Source: CAD feature listing. Evaluate the final solid. Frame: model axes, mm. Face numbers are marked on the shaded views. Round coordinates to 2 decimals unless told otherwise and drop trailing zeros. Order: outer loops, then holes, each group sorted by start corner. A loop starts at its lowest first (then second) coordinate and runs counter-clockwise, first axis right, second up. Notation, with made-up numbers: (-29.75, 83) -> (-22.75, 83) arc R38 cw to (-22.75, 122) -> close; hole circle Ø6 at (-2.5, 54.25). An arc over 180 degrees is marked (long way). Answer as CSV lines item,"result".
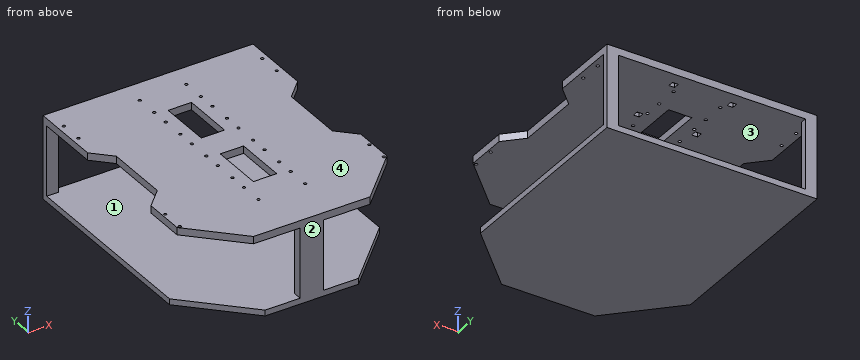
Autodesk Inventor part; units mm, degrees
ref_plane "YZ Plane" through (0, 0, 0) normal (1, 0, 0) x (0, 1, 0)
ref_plane "XZ Plane" through (0, 0, 0) normal (0, 1, 0) x (-1, 0, 0)
ref_plane "XY Plane" through (0, 0, 0) normal (0, 0, 1) x (1, 0, 0)
sketch "Boceto1" plane through (0, 0, 0) normal (0, 0, 1) x (1, 0, 0)
  line L0 (0, 0) -> (-180, 0)
  line L1 (-180, 0) -> (-180, -120)
  line L2 (-180, -120) -> (-150, -150)
  line L3 (-150, -150) -> (-150, -260)
  line L4 (-150, -260) -> (-180, -290)
  line L5 (-180, -290) -> (-180, -360)
  line L6 (-180, -360) -> (-100, -440)
  line L7 (-100, -440) -> (0, -440)
  line L8 (0, -440) -> (0, 0) construction
  line L9 (0, 0) -> (180, 0)
  line L10 (180, 0) -> (180, -120)
  line L11 (180, -120) -> (150, -150)
  line L12 (150, -150) -> (150, -260)
  line L13 (150, -260) -> (180, -290)
  line L14 (180, -290) -> (180, -360)
  line L15 (180, -360) -> (100, -440)
  line L16 (100, -440) -> (0, -440)
  dimension "d0" = 120
  dimension "d1" = 70
  dimension "d2" = 110
  dimension "d3" = 180
  dimension "d8" = 100
  dimension "d9" = 80
  dimension "d13" = 150
  dimension "d17" = 80
  dimension "d18" = 30
  dimension "d19" = 30
extrude "Extrusión1" add sketch "Boceto1" along normal mid plane 12.55
sketch "Boceto2" plane through (0, 0, 6.275) normal (0, 0, 1) x (1, 0, 0)
  line L0 (0, 0) -> (0, -440)
  line L1 (-100, -440) -> (100, -440)
  line L2 (180, 0) -> (180, -120)
  line L3 (180, -120) -> (-179.9429, -120)
  line L4 (180, -120) -> (150, -150)
  line L5 (180, -120) -> (180, -60)
  line L6 (180, -60) -> (0, -60)
  line L7 (0, -60) -> (15, -60)
  line L8 (15, -60) -> (-15, -60)
  line L9 (180, -60) -> (170, -60)
  line L10 (170, -60) -> (170, -79.5)
  line L11 (170, -79.5) -> (170, -40.5)
  circle A0 centre (170, -40.5) radius 2.5
  circle A1 centre (170, -79.5) radius 2.5
  circle A2 centre (-170, -40.5) radius 2.5
  circle A3 centre (-170, -79.5) radius 2.5
  dimension "d20" = 60
  dimension "d22" = 30
  dimension "d23" = 10
  dimension "d25" = 39
  dimension "d26" = 5
extrude "Extrusión2" cut sketch "Boceto2" against normal blind 14.75 contours A1 | A0 | A2 | A3
sketch "Boceto3" plane through (0, 0, 6.275) normal (0, 0, 1) x (1, 0, 0)
  circle A0 centre (170, -40.5) radius 2.5
  line L0 (170, -40.5) -> (170, -60)
  line L1 (170, -60) -> (0, -60)
  line L2 (0, -60) -> (0, -130)
  line L3 (0, -130) -> (40, -130)
  line L4 (40, -130) -> (-40, -130)
  line L5 (40, -130) -> (40, -110.5)
  circle A1 centre (40, -110.5) radius 2.5
  circle A2 centre (40, -149.5) radius 2.5
  circle A3 centre (-40, -110.5) radius 2.5
  circle A4 centre (-40, -149.5) radius 2.5
  line L6 (40, -130) -> (40, -200)
  line L7 (40, -200) -> (40, -165)
  line L8 (40, -165) -> (-88.7042, -165)
  circle A5 centre (40, -219.5) radius 2.5
  circle A6 centre (40, -180.5) radius 2.5
  circle A7 centre (-40, -219.5) radius 2.5
  circle A8 centre (-40, -180.5) radius 2.5
  line L9 (40, -180.5) -> (40, -200)
  line L10 (40, -200) -> (40, -270)
  line L11 (40, -270) -> (-42.5, -270)
  line L12 (40, -270) -> (40, -235)
  line L13 (40, -235) -> (-24.3521, -235)
  circle A9 centre (40, -359.5) radius 2.5
  circle A10 centre (40, -320.5) radius 2.5
  circle A11 centre (-40, -359.5) radius 2.5
  circle A12 centre (-40, -320.5) radius 2.5
  circle A13 centre (40, -250.5) radius 2.5
  circle A14 centre (40, -289.5) radius 2.5
  circle A15 centre (-40, -250.5) radius 2.5
  circle A16 centre (-40, -289.5) radius 2.5
  line L14 (40, -165) -> (40, -95)
  line L15 (40, -95) -> (-4.3592, -95)
  circle A17 centre (40, -79.5) radius 2.5
  circle A18 centre (40, -40.5) radius 2.5
  circle A19 centre (-40, -79.5) radius 2.5
  circle A20 centre (-40, -40.5) radius 2.5
  point P0 (0, 0)
  dimension "d29" = 19.5
  dimension "d30" = 70
  dimension "d31" = 40
  dimension "d32" = 80
  dimension "d33" = 19.5
  dimension "d34" = 5
  dimension "d37" = 70
  dimension "d38" = 70
  dimension "d39" = 35
  dimension "d46" = 70
extrude "Extrusión3" cut sketch "Boceto3" against normal blind 14.75 contours A13 L10 | L10 A13 | A5 L10 | L10 A5 | A6 L6 | L6 A6 | A2 L6 | L6 A2 | L14 L5 A1 | A1 L5 L14 | A3 | A4 | A7 | A8 | A9 | A10 | A11 | A12 | A14 | A15 | A16 | A17 | A18 | A19 | A20
sketch "Boceto4" plane through (0, 0, 6.275) normal (0, 0, 1) x (1, 0, 0)
  circle A0 centre (40, -320.5) radius 2.5
  line L0 (40, -320.5) -> (180, -320.5)
  line L1 (180, -360) -> (180, -290)
  line L2 (180, -320.5) -> (175, -320.5)
  line L3 (175, -320.5) -> (175, -359.5)
  circle A1 centre (175, -320.5) radius 2.5
  circle A2 centre (175, -359.5) radius 2.5
  line L4 (-100, -440) -> (100, -440)
  line L5 (0, -440) -> (0, 0)
  circle A3 centre (-175, -320.5) radius 2.5
  circle A4 centre (-175, -359.5) radius 2.5
  dimension "d40" = 5
  dimension "d41" = 39
  dimension "d42" = 5
  dimension "d43" = 5
extrude "Extrusión4" cut sketch "Boceto4" against normal blind 14.75 contours A2 | A1 L0 | L0 L3 A1 | L0 A1 L3 | A3 | A4
sketch "Boceto6" plane through (0, 0, -6.275) normal (0, 0, -1) x (-1, 0, 0)
  circle A0 centre (40, -289.5) radius 2.5
  circle A1 centre (-40, -289.5) radius 2.5
  line L0 (40, -289.5) -> (-40, -289.5)
  circle A2 centre (-40, -250.5) radius 2.5
  line L1 (-40, -289.5) -> (-40, -250.5)
  circle A3 centre (40, -250.5) radius 2.5
  line L2 (-40, -250.5) -> (40, -250.5)
  line L3 (40, -250.5) -> (40, -289.5)
  line L4 (0, -289.5) -> (20, -289.5)
  line L5 (20, -289.5) -> (20, -250.5)
  line L6 (20, -250.5) -> (-20, -250.5)
  line L7 (-20, -250.5) -> (-20, -289.5)
  line L8 (20, -289.5) -> (20, -314.5)
  line L9 (20, -314.5) -> (-20, -314.5)
  line L10 (-20, -314.5) -> (-20, -289.5)
  line L11 (20, -250.5) -> (20, -225.5)
  line L12 (20, -225.5) -> (-20, -225.5)
  line L13 (-20, -225.5) -> (-20, -250.5)
  point P0 (0, 0)
  dimension "d56" = 40
  dimension "d57" = 25
  dimension "d58" = 25
extrude "Extrusión6" cut sketch "Boceto6" against normal blind 14.75 contours L8 L9 L10 L0 | L0 L7 L2 L5 | L2 L13 L12 L11
sketch "Boceto7" plane through (0, 0, -6.275) normal (0, 0, -1) x (-1, 0, 0)
  circle A0 centre (40, -110.5) radius 2.5
  circle A1 centre (-40, -110.5) radius 2.5
  line L0 (40, -110.5) -> (-40, -110.5)
  circle A2 centre (-40, -149.5) radius 2.5
  line L1 (-40, -110.5) -> (-40, -149.5)
  line L2 (-40, -149.5) -> (40, -149.5)
  line L3 (40, -149.5) -> (40, -110.5)
  line L4 (0, -149.5) -> (-20, -149.5)
  line L5 (-20, -149.5) -> (20, -149.5)
  line L6 (20, -149.5) -> (20, -110.5)
  line L7 (20, -149.5) -> (20, -174.5)
  line L8 (20, -174.5) -> (-20, -174.5)
  line L9 (-20, -174.5) -> (-20, -149.5)
  line L10 (20, -110.5) -> (20, -85.5)
  line L11 (20, -85.5) -> (-20, -85.5)
  line L12 (-20, -85.5) -> (-20, -110.5)
  line L13 (-20, -149.5) -> (-20, -110.5)
  point P0 (0, 0)
  dimension "d63" = 25
  dimension "d64" = 40
  dimension "d65" = 25
  dimension "d66" = 40
extrude "Extrusión7" cut sketch "Boceto7" against normal blind 14.75 contours L6 L2 L13 L0 | L0 L12 L11 L10 | L7 L8 L9 L2
sketch "Boceto8" plane through (0, 0, -6.275) normal (0, 0, -1) x (-1, 0, 0)
  line L0 (0, 0) -> (0, -20)
  line L1 (0, -20) -> (-45, -20)
  line L2 (-45, -20) -> (45, -20)
  line L3 (45, -20) -> (45, -30)
  line L4 (45, -30) -> (55, -30)
  line L5 (55, -30) -> (55, -20)
  line L6 (55, -20) -> (45, -20)
  line L7 (-45, -20) -> (-45, -30)
  line L8 (-45, -30) -> (-55, -30)
  line L9 (-55, -30) -> (-55, -20)
  line L10 (-55, -20) -> (-45, -20)
  line L11 (55, -30) -> (55, -115)
  line L12 (55, -115) -> (45, -115)
  line L13 (45, -115) -> (45, -125)
  line L14 (45, -125) -> (55, -125)
  line L15 (55, -125) -> (55, -115)
  line L16 (-45, -30) -> (-45, -115)
  line L17 (-45, -115) -> (-55, -115)
  line L18 (-55, -115) -> (-55, -125)
  line L19 (-55, -125) -> (-45, -125)
  line L20 (-45, -125) -> (-45, -115)
  dimension "d69" = 20
  dimension "d70" = 45
  dimension "d71" = 90
  dimension "d72" = 10
  dimension "d73" = 10
  dimension "d74" = 10
  dimension "d75" = 10
  dimension "d76" = 10
  dimension "d77" = 10
  dimension "d78" = 85
  dimension "d79" = 10
  dimension "d80" = 10
  dimension "d81" = 10
  dimension "d82" = 85
  dimension "d83" = 10
  dimension "d84" = 10
  dimension "d85" = 10
extrude "Extrusión8" cut sketch "Boceto8" against normal blind 7
sketch "Boceto9" plane through (0, 0, -6.275) normal (0, 0, -1) x (-1, 0, 0)
  line L0 (180, -120) -> (180, 0)
  line L1 (180, 0) -> (180, -10)
  line L2 (180, -10) -> (160, -10)
  line L3 (160, -10) -> (160, 0)
  line L4 (-180, 0) -> (180, 0)
  line L5 (-180, 0) -> (-180, -10)
  line L6 (-180, 0) -> (-180, -120)
  line L7 (-180, -10) -> (-160, -10)
  line L8 (-160, -10) -> (-160, 0)
  line L9 (-160, 0) -> (-180, 0)
  line L10 (160, 0) -> (180, 0)
  point P0 (0, 0)
  dimension "d88" = 10
  dimension "d89" = 20
  dimension "d90" = 10
  dimension "d91" = 20
extrude "Extrusión9" add sketch "Boceto9" along normal blind 130
sketch "Boceto10" plane through (-160, -10, -6.275) normal (1, 0, 0) x (0, 0, -1)
  line L0 (0, 10) -> (130, 10)
  line L1 (130, 10) -> (130, 0)
  line L2 (130, 10) -> (130, 0)
  line L3 (130, 0) -> (120, 0)
  line L4 (0, 0) -> (130, 0)
  line L5 (120, 0) -> (120, 10)
  line L6 (120, 10) -> (130, 10)
  point P0 (-6.275, 10)
  dimension "d94" = 10
  dimension "d95" = 10
extrude "Extrusión10" add sketch "Boceto10" along normal blind 320
sketch "Boceto11" plane through (160, -10, -6.275) normal (0, -1, 0) x (1, 0, 0)
  line L0 (0, 0) -> (0, -120)
  line L1 (0, -120) -> (20, -120)
  line L2 (20, 0) -> (20, -130)
  line L3 (-340, 0) -> (-340, -130)
  line L4 (-320, 0) -> (-320, -120)
  line L5 (-340, -120) -> (-320, -120)
  line L6 (20, -130) -> (-340, -130)
  line L7 (-320, -120) -> (0, -120)
  line L8 (-340, -120) -> (0, -120)
  line L9 (0, -120) -> (20, -120)
  point P0 (-160, 6.275)
extrude "Extrusión11" add sketch "Boceto11" along normal blind 430
chamfer "Chaflán1" distance 100 angle 45 2 edges at (180, -440, -131.275) (-180, -440, -131.275)
sketch "Boceto12" plane through (0, 0, -6.275) normal (0, 0, -1) x (-1, 0, 0)
  line L0 (-100, -440) -> (100, -440)
  line L1 (0, -440) -> (20, -440)
  line L2 (20, -440) -> (-20, -440)
  line L3 (-20, -440) -> (-20, -425)
  line L4 (-20, -425) -> (20, -425)
  line L5 (20, -425) -> (20, -440)
  point P0 (0, 0)
  dimension "d103" = 20
  dimension "d104" = 40
  dimension "d105" = 15
  dimension "d106" = 40
extrude "Extrusión12" add sketch "Boceto12" along normal blind 125
properties part number "BaseCarro" material "Balsa"
1. Line query: L1, parallel to X at y = -40, z = -2; L2, parallel to Z at x = -102, y = -93.5 (3 decimals); L3, parallel to X at y = -359.5, z = 3. Output: solid intervals per line, ascending. Write a range as [from, to].
Results below:
L1,"[-180, -172.45], [-167.55, -42.45], [-37.55, 37.55], [42.45, 167.55], [172.45, 180]"
L2,"[-136.275, -126.275], [-6.275, 6.275]"
L3,"[-180, -177.5], [-172.5, -42.5], [-37.5, 37.5], [42.5, 172.5], [177.5, 180]"
2. Section query D-D on z = -41.5. Return loops of the section in (x, y), and give its area (3 significant figures).
Results below:
outline,"(-180, -10) -> (-160, -10) -> (-160, 0) -> (-180, 0) -> close; (-20, -440) -> (20, -440) -> (20, -425) -> (-20, -425) -> close; (160, -10) -> (180, -10) -> (180, 0) -> (160, 0) -> close"
area,"1,000 mm2"
3. Section query C-C on y = -55. Return loops of the section in (x, z) (3 decimals).
Results below:
outline,"(-180, -136.275) -> (180, -136.275) -> (180, -126.275) -> (-180, -126.275) -> close; (-180, -6.275) -> (180, -6.275) -> (180, 6.275) -> (-180, 6.275) -> close"
4. Pin query (flat end, axial travel): pin 1 (3 mm diameter, centred on x = 40, y = -180.5, fed in from +Z) (3 decimals); pin 2 (14 mm diameter, centred on y = -187.5, z = 0.5, fed in from +X); pin 3 (14 mm diameter, centred on y = -149, z = -0.5, fed in from -X). Return the tip coordinate at first contact, or that it passes through.
Results below:
pin 1,"z = -126.275"
pin 2,"x = 150"
pin 3,"x = -158"
5. Mould query, pull axis Z, two halves, no side actions, for the marked faces 1, 2, 3 and 4. Classes: released by +Z, released by -Z, zero draft, split by the parting line, or undercut.
Results below:
face 1,"undercut"
face 2,"zero draft"
face 3,"undercut"
face 4,"released by +Z"
6. Section query A-A on x = 86.5. Return loops of the section in (y, z) (3 decimals).
Results below:
outline,"(-440, -6.275) -> (0, -6.275) -> (0, 6.275) -> (-440, 6.275) -> close; (-433.5, -136.275) -> (0, -136.275) -> (0, -126.275) -> (-433.5, -126.275) -> close"
7. Section query B-B on x = -12. Return loops of the section in (y, z) (3 decimals), and give its area (3 significant figures).
Results below:
outline,"(-440, -136.275) -> (0, -136.275) -> (0, -126.275) -> (-425, -126.275) -> (-425, -6.275) -> (-314.5, -6.275) -> (-314.5, 6.275) -> (-440, 6.275) -> close; (-225.5, -6.275) -> (-174.5, -6.275) -> (-174.5, 6.275) -> (-225.5, 6.275) -> close; (-85.5, -6.275) -> (0, -6.275) -> (0, 6.275) -> (-85.5, 6.275) -> close"
area,"9,490 mm2"
